For this review, take the finished solid that the model builds, in its own axes (mm). A direction names the side the tool comes from. Round coordinates to 2 decimals unless told otherwise and drop trailing zeros. Write each loop counter-clockwise with the first axis right and the second up, starting at its lowest first coordinate (ties: lowest second). Pieces come first, ordered by that corner, then holes. Notation, with made-up numbers: (59, 73) -> (74, 73) arc R13 cw to (74, 94) -> close; hole circle Ø8 at (3, 22). An arc over 180 degrees is marked (long way). Answer in a Markdown table with one row per item.
from build123d import *

# Parameters (mm, degrees)
EXTRUDE_1_DEPTH     = 20
CUT_EXTRUDE_START   = 30
SKETCH_2_W          = 17.5
SKETCH_2_H          = 16.6
CUT_EXTRUDE_1_DEPTH = 27.5
CUT_EXTRUDE_START_2 = 17.5
SKETCH_3_R          = 2
CUT_EXTRUDE_2_DEPTH = 2.5
CUT_EXTRUDE_3_REACH = 43.231
SKETCH_4_R          = 1.7


with BuildPart() as part:
    # 草图1 → 凸台-拉伸1 (new body)
    with BuildSketch(Plane.XY):
        Polygon((0, 0), (20, 0), (20, 30), (17.5, 30), (0, 2.5), align=None)
    extrude(amount=-EXTRUDE_1_DEPTH)

    # 草图2 → 切除-拉伸1 (cut)
    with BuildSketch(Plane(origin=(0, 0, 0), x_dir=(1, 0, 0), z_dir=(0, 1, 0)).offset(CUT_EXTRUDE_START)):
        with Locations((8.75, 10)):
            Rectangle(SKETCH_2_W, SKETCH_2_H)
    extrude(amount=-CUT_EXTRUDE_1_DEPTH, mode=Mode.SUBTRACT)

    # 草图3 → 切除-拉伸2 (cut)
    with BuildSketch(Plane(origin=(0, 0, 0), x_dir=(0, 0, -1), z_dir=(1, 0, 0)).offset(CUT_EXTRUDE_START_2)):
        with Locations(Location((10, 22, 0), (0, 0, 180))):
            Circle(SKETCH_3_R)
        with Locations(Location((10, 10, 0), (0, 0, 180))):
            Circle(SKETCH_3_R)
    extrude(amount=CUT_EXTRUDE_2_DEPTH, mode=Mode.SUBTRACT)

    # 草图4 → 切除-拉伸3 (cut, up to next)
    with BuildSketch(Plane(origin=(0, 0, 0), x_dir=(1, 0, 0), z_dir=(0, 1, 0)), mode=Mode.PRIVATE) as cut_extrude_3_sk1:
        with Locations(Location((9, 10, 0), (0, 0, 90))):
            Circle(SKETCH_4_R)
    cut_extrude_3_tool1 = extrude(cut_extrude_3_sk1.sketch, amount=CUT_EXTRUDE_3_REACH, mode=Mode.PRIVATE) & part.part
    add(cut_extrude_3_tool1.solids().sort_by_distance((9, 0, -10))[0], mode=Mode.SUBTRACT)


solid = part.part
1) Mouldability with a two-part tool opening along Z and no side actions: class faces 3 (the flat face through (12, 12, 0)), 4 (the flat face through (12, 0, -10)), 5 (the flat face through (9, 2.5, -12)) as pulls with the +Z half, pulls with the -Z half, needs draft (parallel to the pull), parting line crosses it, or undercut.
Solved:
| item | result |
|---|---|
| face 3 | pulls with the +Z half |
| face 4 | needs draft |
| face 5 | undercut |
2) For line 1 (Y direction, x = 18.25, z = -10); line 2 (Z direction, x = 18.9, y = 10); line 3 (Z direction, x = 9, y = 1.8), list the stretches that pass through material, from the lowest coordinate up. Write a range as [from, to].
Solved:
| item | result |
|---|---|
| line 1 | [0, 8], [12, 20], [24, 30] |
| line 2 | [-20, -12], [-8, 0] |
| line 3 | [-20, -11.7], [-8.3, 0] |
3) Consider section C-C on y = 10. State the section outline as (x, z) points, then the cut area to 3 significant figures.
Solved:
| item | result |
|---|---|
| outline | (4.77, -20) -> (20, -20) -> (20, -12) -> (17.5, -12) -> (17.5, -18.3) -> (4.77, -18.3) -> close; (4.77, -1.7) -> (17.5, -1.7) -> (17.5, -8) -> (20, -8) -> (20, 0) -> (4.77, 0) -> close |
| area | 83.3 mm² |
4) Consider section B-B on x = 3.5. State the section outline as (y, z) points, then the cut area to 3 significant figures.
Solved:
| item | result |
|---|---|
| outline | (0, -20) -> (8, -20) -> (8, -18.3) -> (2.5, -18.3) -> (2.5, -1.7) -> (8, -1.7) -> (8, 0) -> (0, 0) -> close |
| area | 68.7 mm² |
5) Consider section A-A on z = -10. State the section outline as (x, y) points.
Solved:
| item | result |
|---|---|
| outline | (0, 0) -> (7.3, 0) -> (7.3, 2.5) -> (0, 2.5) -> close; (10.7, 0) -> (20, 0) -> (20, 8) -> (17.5, 8) -> (17.5, 2.5) -> (10.7, 2.5) -> close; (17.5, 12) -> (20, 12) -> (20, 20) -> (17.5, 20) -> close; (17.5, 24) -> (20, 24) -> (20, 30) -> (17.5, 30) -> close |
6) Clearance check with flat-ended pins moving along their axes: pin 1 Ø12 at (y, z) = (7.5, -5.5) entering from -X; pin 2 Ø1.5 at (x, z) = (12, -4) entering from +Y; pin 3 Ø5 at (y, z) = (19.5, -7) entering from -X; pin 4 Ø2 at (x, z) = (14, -18) entering from +Y. State where each tip first meets the part, or that it passes through.
Solved:
| item | result |
|---|---|
| pin 1 | x = 0 |
| pin 2 | y = 2.5 |
| pin 3 | x = 17.5 |
| pin 4 | y = 26 |
7) Consider section D-D on x = 9. State the section outline as (y, z) points.
Solved:
| item | result |
|---|---|
| outline | (0, -20) -> (16.64, -20) -> (16.64, -18.3) -> (2.5, -18.3) -> (2.5, -11.7) -> (0, -11.7) -> close; (0, -8.3) -> (2.5, -8.3) -> (2.5, -1.7) -> (16.64, -1.7) -> (16.64, 0) -> (0, 0) -> close |
8) For faces 1 (the flat face through (13, 10, -1.7)), 2 (the flat face through (8.87, 16.44, -0.84)), list the 3-axis set-ups (+Z, -Z, +X, -X, +Y, -Y) from which the entire face can be reached by the end or side of a thin tool; tool diameter is ignored.
Solved:
| item | result |
|---|---|
| face 1 | -X, +Y |
| face 2 | +Z, -Z, -X, +Y |
